Could you check a few things on this model? Use its own coordinates, in mm. A direction names the side the tool comes from. Round coordinates to 2 decimals unless told otherwise and drop trailing zeros. Write each loop counter-clockwise with the first axis right and the second up, starting at its lowest first coordinate (ties: lowest second). Pieces come first, ordered by that corner, then holes. Notation, with made-up numbers: M -6.75,-2.75 L 31.25,-2.75 A9 ccw 31.25,2.25 Z; hole C 14,74 d9. An arc over 180 degrees is marked long. One line per item, written item: value. Start each with the question number.
(1) I want a section at A-A on z = 15. Please give me the cut outline in (x, y), and give its area (3 significant figures).
(2) I want a section at B-B on y = 54. Please give me the cut outline in (x, z).
(3) I'm going to push flat-ended pins straight in: pin 1 Ø1.5 at (x, y) = (79, 37) entering from -Z; pin 2 Ø5 at (x, z) = (46.5, 16) entering from -Y; pin 3 Ø3 at (y, z) = (-35, 14) entering from +X; pin 4 Ø3 at (y, z) = (-32, 15) entering from -X. Where does each tip first touch, or does it pass through?
(4) Thinking about a two-plate mould opening in X: for faces 3 (the face through (116, -2, 16)), 4 (the face through (-2, 120, 6)), 5 (the face through (110, -2, 15)), 6 (the face through (-120, -2, 6)), which applies, released by +X, released by -X, zero draft, split by the parting line, or undercut?
(5) If I drill on L1, parallel to Y at x = 27.5, z = 10.75; L2, parallel to X at y = 75.5, z = 13.75; L3, parallel to X at y = 31, z = 16.75, over which ranges is the centre line in solid material (lowest first)?
(6) Which directions (+Z, -Z, +X, -X, +Y, -Y) give clear straight access to the entire face, cutting with the end or side of a thin tool? Please do faces 1 (the face through (-2, 110, 15)), 2 (the face through (120, -2, 6)).
```python
from build123d import *

# Parameters (mm, degrees)
SKETCH_1_W          = 240
SKETCH_1_H          = 240
EXTRUDE_1_DEPTH     = 20
CHAMFER_1_SIZE      = 8
SKETCH_2_W          = 220
SKETCH_2_H          = 220
SKETCH_2_W_2        = 200
SKETCH_2_H_2        = 200
CUT_EXTRUDE_1_DEPTH = 10


with BuildPart() as part:
    # Эскиз1 → Бобышка-Вытянуть1 (new body)
    with BuildSketch(Plane.XY):
        Rectangle(SKETCH_1_W, SKETCH_1_H)
    extrude(amount=EXTRUDE_1_DEPTH)

    # Фаска1
    chamfer_1_edges = [part.edges().sort_by_distance(p)[0] for p in [
        (0, -120, 20),
        (-120, 0, 20),
        (0, 120, 20),
        (120, 0, 20),
    ]]
    chamfer(chamfer_1_edges, length=CHAMFER_1_SIZE)

    # Эскиз2 → Вырез-Вытянуть1 (cut)
    with BuildSketch(Plane.XY.offset(20)):
        Rectangle(SKETCH_2_W, SKETCH_2_H)
        Rectangle(SKETCH_2_W_2, SKETCH_2_H_2, mode=Mode.SUBTRACT)
    extrude(amount=-CUT_EXTRUDE_1_DEPTH, mode=Mode.SUBTRACT)


solid = part.part
```
Found:
1. outline: M -117,-117 L 117,-117 L 117,117 L -117,117 Z; M -100,-100 L 100,-100 L 100,100 L -100,100 Z; hole M -110,-110 L 110,-110 L 110,110 L -110,110 Z
1. area: 46,400 mm²
2. outline: M -120,0 L 120,0 L 120,12 L 112,20 L 110,20 L 110,10 L 100,10 L 100,20 L -100,20 L -100,10 L -110,10 L -110,20 L -112,20 L -120,12 Z
3. pin 1: stops at z = 0
3. pin 2: stops at y = -118.5
3. pin 3: stops at x = 119.5
3. pin 4: stops at x = -118.5
4. face 3: released by +X
4. face 4: zero draft
4. face 5: undercut
4. face 6: released by -X
5. L1: y = -120 to -110, -100 to 100, 110 to 120
5. L2: x = -118.25 to -110, -100 to 100, 110 to 118.25
5. L3: x = -115.25 to -110, -100 to 100, 110 to 115.25
6. face 1: +Z
6. face 2: +Z, -Z, +X, +Y, -Y
